Here's the drawing with two shaded views (mm, measured from the low corner). I have some questions. A direction names the side the tool comes from. Round coordinates to 2 decimals unless told otherwise and drop trailing zeros. Write each loop counter-clockwise with the first axis right and the second up, starting at its lowest first coordinate (ties: lowest second). Pieces come first, ordered by that corner, then holes. Notation, with made-up numbers: (-31, 79.5) - (-18, 79.5) arc R28 cw to (-18, 100.5) - close; hole circle Ø4 at (80, -1). An arc over 180 degrees is marked (long way). Return JSON: item names as keys, results as strings. Group by question number.
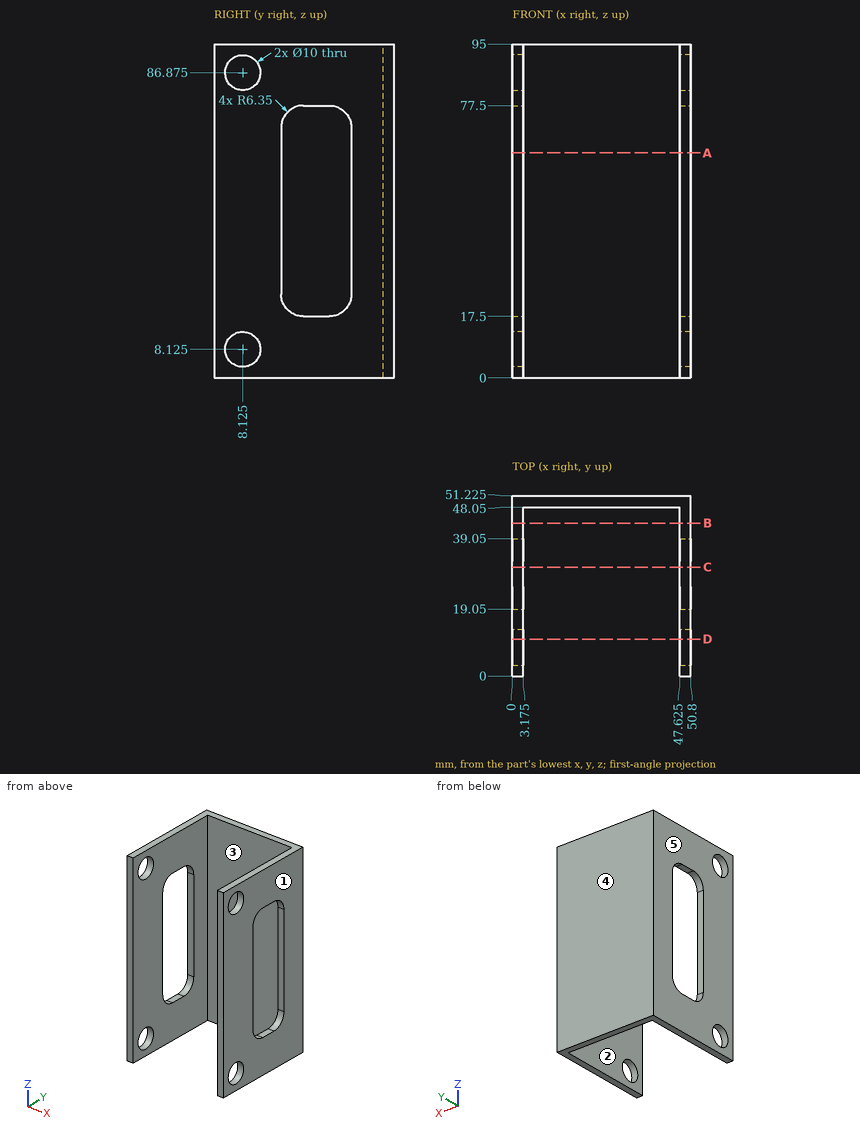
1) For the marked faces 1 and 2, which set-ups out of +Z, -Z, +X, -X, +Y, -Y let a thin tool reach every point of the face, with its end or its side?
2) Imagine slicing it at A-A (z = 64). Please give me the cut outline in (x, y) (3 decimals).
3) Will these pins go through, and if not, where does the flat tip stop? pin 1 Ø8 at (x, z) = (23.5, 11) entering from -Y; pin 2 Ø8 at (y, z) = (8.125, 8.125) entering from -X.
4) I need wall thicknesses on line 1 along X through (y, z) = (41, 60) (3 decimals); line 2 along Y through (x, z) = (21, 6.5) (3 decimals); line 3 along Y through (x, z) = (48.5, 73) (3 decimals). Which ranges of each line are inside material? Lowest first, please.
5) Imagine slicing it at C-C (y = 31). Please give me the cut outline in (x, z) (3 decimals).
6) Imagine slicing it at B-B (y = 43.5). Please give me the cut outline in (x, z) (3 decimals).
7) Imagine slicing it at D-D (y = 10.5). Please give me the cut outline in (x, z) (3 decimals).
8) If we mould it in two halves opening along X, with no side actions, what happens to the marked faces 3, 4 and 5? For each: released by +X, released by -X, zero draft, split by the parting line, or undercut.
Results found:
{
 "1": {"face 1": "+Z, -Z, +X, +Y, -Y", "face 2": "+Z, -Z, -Y"},
 "2": {"outline": "(0, 0) - (3.175, 0) - (3.175, 19.05) - (0, 19.05) - close; (0, 39.05) - (3.175, 39.05) - (3.175, 48.05) - (47.625, 48.05) - (47.625, 39.05) - (50.8, 39.05) - (50.8, 51.225) - (0, 51.225) - close; (47.625, 0) - (50.8, 0) - (50.8, 19.05) - (47.625, 19.05) - close"},
 "3": {"pin 1": "stops at y = 48.05", "pin 2": "passes through"},
 "4": {"line 1": "x = 0 to 3.175, 47.625 to 50.8", "line 2": "y = 48.05 to 51.225", "line 3": "y = 0 to 19.325, 38.775 to 51.225"},
 "5": {"outline": "(0, 0) - (3.175, 0) - (3.175, 17.5) - (0, 17.5) - close; (0, 77.5) - (3.175, 77.5) - (3.175, 95) - (0, 95) - close; (47.625, 0) - (50.8, 0) - (50.8, 17.5) - (47.625, 17.5) - close; (47.625, 77.5) - (50.8, 77.5) - (50.8, 95) - (47.625, 95) - close"},
 "6": {"outline": "(0, 0) - (3.175, 0) - (3.175, 95) - (0, 95) - close; (47.625, 0) - (50.8, 0) - (50.8, 95) - (47.625, 95) - close"},
 "7": {"outline": "(0, 0) - (3.175, 0) - (3.175, 3.725) - (0, 3.725) - close; (0, 12.525) - (3.175, 12.525) - (3.175, 82.475) - (0, 82.475) - close; (0, 91.275) - (3.175, 91.275) - (3.175, 95) - (0, 95) - close; (47.625, 0) - (50.8, 0) - (50.8, 3.725) - (47.625, 3.725) - close; (47.625, 12.525) - (50.8, 12.525) - (50.8, 82.475) - (47.625, 82.475) - close; (47.625, 91.275) - (50.8, 91.275) - (50.8, 95) - (47.625, 95) - close"},
 "8": {"face 3": "undercut", "face 4": "zero draft", "face 5": "released by -X"}
}
